Check sheet for the modelled part. Datum: model origin and axes. Units: mm. Face numbers are marked on the shaded views. A direction names the side the tool comes from. Round coordinates to 2 decimals unless told otherwise and drop trailing zeros. Loops run counter-clockwise (first coordinate to the right, second up) from the corner with the lowest first, then second, coordinate; pieces in that order, holes last. Notation, with made-up numbers: (-13.5, 87) - (10.5, 87) arc R24 ccw to (10.5, 102) - close; hole circle Ø9 at (88.5, 21.5). An arc over 180 degrees is marked (long way). Return JSON: item names as keys, results as strings.
Autodesk Inventor part; units mm, degrees
ref_plane "YZ Plane" through (0, 0, 0) normal (1, 0, 0) x (0, 1, 0)
ref_plane "XZ Plane" through (0, 0, 0) normal (0, 1, 0) x (-1, 0, 0)
ref_plane "XY Plane" through (0, 0, 0) normal (0, 0, 1) x (1, 0, 0)
sketch "Sketch1" plane through (0, 0, 0) normal (0, 0, 1) x (1, 0, 0)
  line L0 (-98.4355, -21.9546) -> (-43.0099, 10.0454)
  line L1 (-43.0099, 10.0454) -> (-24.0099, -22.8636)
  line L2 (-24.0099, -22.8636) -> (-79.4355, -54.8636)
  line L3 (-79.4355, -54.8636) -> (-98.4355, -21.9546)
  line L4 (-6.35, -7.3) -> (0, -7.3)
  line L5 (0, -7.3) -> (0, -13.65)
  line L6 (0, -13.65) -> (-6.35, -13.65)
  line L7 (-6.35, -13.65) -> (-6.35, -7.3)
  line L8 (6.35, -4.953) -> (0, -4.953)
  line L9 (0, -4.953) -> (0, 4.953)
  line L10 (0, 4.953) -> (6.35, 4.953)
  line L11 (6.35, 4.953) -> (6.35, -4.953)
  line L12 (-6.35, 13.65) -> (0, 13.65)
  line L13 (0, 13.65) -> (0, 7.3)
  line L14 (0, 7.3) -> (-6.35, 7.3)
  line L15 (-6.35, 7.3) -> (-6.35, 13.65)
  line L16 (0, -20) -> (-19.05, -20)
  line L17 (-19.05, -20) -> (-19.05, 20)
  line L18 (-19.05, 20) -> (0, 20)
  line L19 (0, 20) -> (0, -20)
  line L20 (-10.9985, -26.35) -> (-39.5235, 23.0567)
  line L21 (-39.5235, 23.0567) -> (-111.4469, -18.4683)
  line L22 (-111.4469, -18.4683) -> (-82.9219, -67.875)
  line L23 (-82.9219, -67.875) -> (-10.9985, -26.35)
  line L24 (-10.9985, -26.35) -> (0, -20)
  line L25 (-19.05, 20) -> (-39.5235, 23.0567)
  point P0 (0, 0)
  point P1 (0, 0)
  dimension "d0" = 6.35
  dimension "d2" = 9.906
  dimension "d3" = 40
  dimension "d4" = 6.35
  dimension "d5" = 6.35
  dimension "d6" = 6.35
  dimension "d7" = 38
  dimension "d8" = 64
  dimension "d9" = 9.525
  dimension "d10" = 30
  dimension "d11" = 19.05
  dimension "d12" = 12.7
extrude "Extrusion1" add sketch "Sketch1" along normal blind 6.35 contours L7 L6 L19 L16 L20 L17 L18 L12 L15 L14 L9 L4 | L9 L10 L11 L8 | L24 L20 L16 | L20 L23 L22 L21 L17 L16 | L16 L17 L20 | L20 L25 L17
properties part number "acrylic kinect bracket"
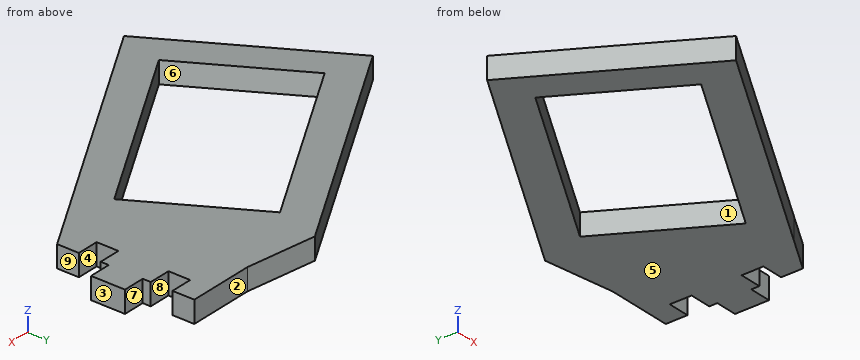
Q1. Sectioned sample at C-C (x = -47.5). Enter the section's corners in (y, z).
Answer key:
{"outline": "(-47.42, 0) - (-36.43, 0) - (-36.43, 6.35) - (-47.42, 6.35) - close; (7.45, 0) - (18.45, 0) - (18.45, 6.35) - (7.45, 6.35) - close"}
Q2. Sectioned sample at B-B (y = -9.5). Enter the section's corners in (x, z).
Answer key:
{"outline": "(-95.91, 0) - (-76.86, 0) - (-76.86, 6.35) - (-95.91, 6.35) - close; (-31.73, 0) - (-6.35, 0) - (-6.35, 6.35) - (-31.73, 6.35) - close"}
Q3. Tool access check on the marked faces 1, 2, 3, 4 and 5. Record the directions out of +Z, -Z, +X, -X, +Y, -Y that give a thin tool (end or side, any length) a straight path to the whole face; none if there is none.
Answer key:
{"face 1": "+Z, -Z", "face 2": "+Z, -Z, +X, +Y", "face 3": "+Z, -Z, +X, +Y, -Y", "face 4": "+Z, -Z, +X", "face 5": "-Z, +X, -X, +Y, -Y"}
Q4. Sectioned sample at D-D (x = -16). Enter the section's corners in (y, z), plus the area to 3 significant figures.
Answer key:
{"outline": "(-29.24, 0) - (20, 0) - (20, 6.35) - (-29.24, 6.35) - close", "area": "313 mm²"}
Q5. Depth check by flat-ended pin: P1, Ø3, axis at y = -57, z = 3, coming from the +X side; P2, Ø3, axis at x = -5.5, z = 5.5, coming from the +Y side; P3, Ø1.9, axis at x = 3, z = 3.5, coming from the -Y side. Enter the tip coordinate at first touch or a pass-through.
Answer key:
{"P1": "stops at x = -61.49", "P2": "stops at y = 20", "P3": "stops at y = -4.95"}
Q6. Draft check along Y on the marked faces 6, 7, 8 and 9. Enter one of: released by +Y, released by -Y, zero draft, split by the parting line, or undercut.
Answer key:
{"face 6": "undercut", "face 7": "released by +Y", "face 8": "undercut", "face 9": "zero draft"}
Q7. Scan lines: probe 1 along Y at (x, z) = (-2, 5.5); probe 2 along Y at (x, z) = (-41, 0.5); probe 3 along X at (y, z) = (-34.5, 4.75). Record each from-to range of solid material in increasing order. Write a range as [from, to].
Answer key:
{"probe 1": "y = [-21.15, -13.65], [-7.3, 7.3], [13.65, 20]", "probe 2": "y = [-43.67, -32.67], [6.56, 22.2]", "probe 3": "x = [-102.19, -91.19], [-44.16, -25.11]"}
